Input: part model. Units: mm. Frame: model coordinates. A direction names the side the tool comes from. Give positions to 0.01 mm unless a question says otherwise; leave off trailing zeros. Loops run counter-clockwise (first coordinate to the right, second up) from the corner with the lowest first, then second, coordinate; pieces in that order, holes last. Notation, with made-up numbers: M -36,-23 L -23,-23 A9 ccw -23,-9 Z; hole C 32.25,-37.75 d4. An arc over 180 degrees is marked long. Use CSV: the item, a comma, the result in double quotes. Start each with the question number.
Q1. Material intervals for line 1 along Y through (x, z) = (-18.25, 67.5); line 2 along Z through (x, y) = (-20, -55.5); line 3 along Z through (x, y) = (-18, -88.9), sorted ascending.
Q2. Pin query (flat end, axial travel): pin 1 (11.5 mm diameter, centred on y = -88.9, z = 114.3, fed in from +X); pin 2 (3 mm diameter, centred on x = -9, z = 101, fed in from +Y); pin 3 (3 mm diameter, centred on x = -3, y = -47.5, fed in from +Z); pin 4 (7.5 mm diameter, centred on x = -7, y = -8, fed in from +Z). Return the tip coordinate at first contact, or that it passes through.
Q3. Section A-A, the plane z = 114.3. Output: boundary loops of the cut face in (x, y).
Q4. Section D-D, the plane z = 95.5. Output: boundary loops of the cut face in (x, y), plus the area to 3 significant figures.
Q5. Reachability of faces 1 (the cylindrical face through (-12.88, -87.52, 108.1)), 2 (the cylindrical face through (-12.88, -70.77, 31.13)), 3 (the flat face through (-13, -13, 76.2)) from +Z, -Z, +X, -X, +Y, -Y: full face, straight path, thin tool, end or side. Return the list, or none.
Q6. Section B-B, the plane x = -14.75. Output: boundary loops of the cut face in (y, z), plus the area to 3 significant figures.
Q7. Pull-direction query (Y, two-part tool) for faces 4 (the cylindrical face through (-12.52, -5.73, 5.43)), 5 (the flat face through (-13, -76.2, 85)), 6 (the flat face through (-13, -101.6, 74)), 7 (the flat face through (-13, -51, 25.4)); classes: released by +Y, released by -Y, zero draft, split by the parting line, or undercut.
Q8. Section C-C, the plane y = -88.9. Output: boundary loops of the cut face in (x, z).
from build123d import *

# Parameters (mm, degrees)
F0_W     = 25.4
F0_H     = 25.4
F1_DEPTH = 101.6
F2_W     = 25.4
F2_H     = 25.4
F3_DEPTH = 127
F4_W     = 25.4
F4_H     = 25.4
F5_DEPTH = 76.2
F7_D     = 12.7
F8_R     = 19.05
F9_R     = 19.05
F10_R    = 19.05
F11_R    = 19.05


with BuildPart() as f1:
    # F0 (on Front) → F1 (new body)
    with BuildSketch(Plane.XZ):
        with Locations((-12.7, 12.7)):
            Rectangle(F0_W, F0_H)
    extrude(amount=F1_DEPTH)

    # F2 (on face) → F3 (join)
    with BuildSketch(Plane(origin=(0, 0, 0), x_dir=(1, 0, 0), z_dir=(0, 0, -1))):
        with Locations((-12.7, 88.9)):
            Rectangle(F2_W, F2_H)
    extrude(amount=-F3_DEPTH)

    # F4 (on face) → F5 (join)
    with BuildSketch(Plane(origin=(0, 0, 0), x_dir=(1, 0, 0), z_dir=(0, 0, -1))):
        with Locations((-12.7, 12.7)):
            Rectangle(F4_W, F4_H)
    extrude(amount=-F5_DEPTH)

    # F7 (through all)
    with Locations(Plane.YZ):
        with Locations((-88.9, 114.3)):
            Hole(F7_D / 2)

    # F8
    f8_edges = [f1.edges().sort_by_distance(p)[0] for p in [
        (-12.7, -76.2, 25.4),
    ]]
    fillet(f8_edges, radius=F8_R)

    # F9
    f9_edges = [f1.edges().sort_by_distance(p)[0] for p in [
        (-12.7, -101.6, 0),
    ]]
    fillet(f9_edges, radius=F9_R)

    # F10
    f10_edges = [f1.edges().sort_by_distance(p)[0] for p in [
        (-12.7, 0, 0),
    ]]
    fillet(f10_edges, radius=F10_R)

    # F11
    f11_edges = [f1.edges().sort_by_distance(p)[0] for p in [
        (-12.7, -25.4, 25.4),
    ]]
    fillet(f11_edges, radius=F11_R)


solid = f1.part
A:
1,line 1,"-101.6 to -76.2, -25.4 to 0"
1,line 2,"0 to 25.4"
1,line 3,"1.09 to 107.95, 120.65 to 127"
2,pin 1,"through"
2,pin 2,"y = -76.2"
2,pin 3,"z = 25.4"
2,pin 4,"z = 76.2"
3,outline,"M -25.4,-101.6 L 0,-101.6 L 0,-95.25 L -25.4,-95.25 Z; M -25.4,-82.55 L 0,-82.55 L 0,-76.2 L -25.4,-76.2 Z"
4,outline,"M -25.4,-101.6 L 0,-101.6 L 0,-76.2 L -25.4,-76.2 Z"
4,area,"645 mm^2"
5,face 1,"+X, -X"
5,face 2,"+Z, +X, -X"
5,face 3,"+Z, +X, -X, +Y"
6,outline,"M -101.6,19.05 A19.05 ccw -82.55,0 L -19.05,0 A19.05 ccw 0,19.05 L 0,76.2 L -25.4,76.2 L -25.4,44.45 A19.05 cw -44.45,25.4 L -57.15,25.4 A19.05 cw -76.2,44.45 L -76.2,127 L -101.6,127 Z; hole C -88.9,114.3 d12.7"
6,area,"6,320 mm^2"
7,face 4,"released by +Y"
7,face 5,"undercut"
7,face 6,"released by -Y"
7,face 7,"undercut"
8,outline,"M -25.4,1.09 L 0,1.09 L 0,107.95 L -25.4,107.95 Z; M -25.4,120.65 L 0,120.65 L 0,127 L -25.4,127 Z"
